from build123d import *

# Parameters (mm, degrees)
F1_DEPTH = 19


with BuildPart() as f1:
    # F0 (on Front) → F1 (new body)
    with BuildSketch(Plane.XZ):
        Polygon((11.51464, 37.958085), (-7.48536, 50.485557), (-7.48536, -216.733724), (11.51464, -229.261196), align=None)
    extrude(amount=F1_DEPTH)


with BuildPart() as f2_1:
    # F2: copy of F1
    add(f1.part)


solid = f1.part
The model under review builds one solid part; all positions refer to its coordinate system, in mm. Round coordinates to 2 decimals unless told otherwise and drop trailing zeros. Order: outer loops, then holes, each group sorted by start corner. A loop starts at its lowest first (then second) coordinate and runs counter-clockwise, first axis right, second up. Notation, with made-up numbers: (24.25, -22) -> (81.25, -22) arc R28 cw to (81.25, -2) -> close; hole circle Ø4 at (-27, 74.25). An arc over 180 degrees is marked (long way). Return JSON: item names as keys, results as strings.
1. Take a section at B-B (x = 4). Write out the cut boundary in (y, z).
Answer block:
{"outline": "(-19, -224.31) -> (0, -224.31) -> (0, 42.91) -> (-19, 42.91) -> close"}
2. For L1, parallel to Z at x = 8.5, y = -10.5; L2, parallel to Z at x = 9.5, y = -8.5, list the stretches that pass through material, from the lowest coordinate up. Write a range as [from, to].
Answer block:
{"L1": "z = [-227.27, 39.95]", "L2": "z = [-227.93, 39.29]"}
3. Take a section at A-A (y = -16.25). Write out the cut boundary in (x, z).
Answer block:
{"outline": "(-7.49, -216.73) -> (11.51, -229.26) -> (11.51, 37.96) -> (-7.49, 50.49) -> close"}
4. Insertion check: P1, Ø6, axis at x = 7.5, z = -114.5, coming from the +Y side; P2, Ø6, axis at x = 2, y = -5, coming from the -Z side; P3, Ø5, axis at x = 7, y = -14, coming from the -Z side; P4, Ø8, axis at x = 4, y = -3, coming from the -Z side. Each pin has a flat end and moves straight along its axis. Give the tip position at first contact, or say it passes through.
Answer block:
{"P1": "stops at y = 0", "P2": "stops at z = -224.97", "P3": "stops at z = -227.93", "P4": "stops at z = -226.94"}
